from build123d import *

# Parameters (mm, degrees)
EXTRUDE_3_DEPTH     = 18
SKETCH_2_R          = 1.8
CUT_EXTRUDE_1_DEPTH = 17.325
SKETCH_4_R          = 1.75
EXTRUDE_9_DEPTH     = 5
SKETCH_7_W          = 17.320508076
SKETCH_7_H          = 5
EXTRUDE_10_DEPTH    = 25
FILLET_1_R          = 5
FILLET_2_R          = 5
SKETCH_8_R          = 20
EXTRUDE_11_DEPTH    = 3


with BuildPart() as part:
    # 草图1 → 凸台-拉伸3 (new body)
    with BuildSketch(Plane(origin=(0, 0, 0), x_dir=(1, 0, 0), z_dir=(0, 1, 0))):
        Polygon((10, 0), (5, 8.660254038), (-5, 8.660254038), (-10, 0), (-5, -8.660254038), (5, -8.660254038), align=None)
        Polygon((6.985938257, 0), (3.492969129, 6.05), (-3.492969129, 6.05), (-6.985938257, 0), (-3.492969129, -6.05), (3.492969129, -6.05), align=None, mode=Mode.SUBTRACT)
    extrude(amount=-EXTRUDE_3_DEPTH)

    # 草图2 → 切除-拉伸1 (cut)
    with BuildSketch(Plane(origin=(7.5, 0, -4.330127019), x_dir=(-0.5000000000000003, 0, -0.8660254037844386), z_dir=(0.8660254037844386, 0, -0.5000000000000003))):
        with Locations((0, -4.5)):
            Circle(SKETCH_2_R)
    extrude(amount=-CUT_EXTRUDE_1_DEPTH, mode=Mode.SUBTRACT)

    # 草图4 → 凸台-拉伸9 (add)
    with BuildSketch(Plane.XZ.offset(18)):
        Polygon((-10, 0), (5, -8.660254038), (10, 0), (5, 8.660254038), (-5, 8.660254038), align=None)
        with Locations(Location((0, 0, 0), (0, 0, 270))):
            Circle(SKETCH_4_R, mode=Mode.SUBTRACT)
    extrude(amount=EXTRUDE_9_DEPTH)

    # 草图7 → 凸台-拉伸10 (add)
    with BuildSketch(Plane(origin=(-2.5, 0, -4.330127019), x_dir=(-0.8660254037844388, 0, 0.49999999999999983), z_dir=(-0.4999999999999998, 0, -0.8660254037844387))):
        with Locations((0, -20.5)):
            Rectangle(SKETCH_7_W, SKETCH_7_H)
    extrude(amount=EXTRUDE_10_DEPTH)

    # 圆角1
    fillet_1_edges = [part.edges().sort_by_distance(p)[0] for p in [
        (-7.5, -20.5, -30.310889132),
    ]]
    fillet(fillet_1_edges, radius=FILLET_1_R)

    # 圆角2
    fillet_2_edges = [part.edges().sort_by_distance(p)[0] for p in [
        (-22.5, -20.5, -21.650635095),
    ]]
    fillet(fillet_2_edges, radius=FILLET_2_R)

    # 草图8 → 凸台-拉伸11 (add)
    with BuildSketch(Plane.XZ.offset(23)):
        with Locations(Location((-12.169872981, -21.078838325, 0), (0, 0, 85.658906273))):
            Circle(SKETCH_8_R)
    extrude(amount=EXTRUDE_11_DEPTH)


solid = part.part
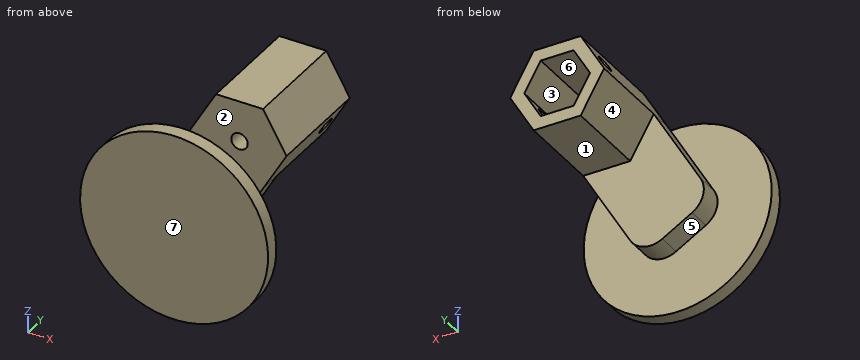
Input: part model. Units: mm. Frame: model coordinates. Face numbers are marked on the shaded views. A direction names the side the tool comes from. Give positions to 0.01 mm unless a question says otherwise; leave off trailing zeros. Write each loop counter-clockwise with the first axis right and the second up, starting at its lowest first coordinate (ties: lowest second). Pieces come first, ordered by that corner, then holes. Notation, with made-up numbers: M 13,35.25 L 64,35.25 A14 cw 64,48.25 Z; hole C 5,-37.5 d4. An arc over 180 degrees is marked long. Write item = value, one per line. Start each with the question number.
1) Draft query along X for the marked faces 5, 6 and 7. Return one class per face: +X half, -X half, draft (parallel to the pull), parting line (faces both ways), or undercut.
2) Reachability of the marked faces 1, 2, 3 and 4 from +Z, -Z, +X, -X, +Y, -Y: full face, straight path, thin tool, end or side. Return the list, or none.
3) First-contact query: pin 1 Ø5 at (x, z) = (-10.5, -22.5) entering from +Y; pin 2 Ø5.5 at (x, y) = (0, -13) entering from -Z; pin 3 Ø1.5 at (y, z) = (-20, -16.5) entering from +X. Flat tips, straight axial feed; report the tip coordinate or a pass-through.
4) Cut plane D-D on x = -26. Return the cut outline in (y, z), then the cut area to 3 significant figures.
5) Cut plane C-C on z = -14. Return the cut outline in (x, y), then the cut area to 3 significant figures.
6) Cut plane A-A on y = -11.5. Return the cut outline in (x, z).
7) Material intervals for line 1 along X through (y, z) = (-19.7, 0); line 2 along Z through (x, y) = (-3, -3.75); line 3 along Y through (x, z) = (-19, -10), sorted ascending. Write a range as [from, to].
8) Cut plane B-B on x = 0. Return the cut outline in (y, z), then the cut area to 3 significant figures.
Solved:
q1.face_5 = -X half
q1.face_6 = undercut
q1.face_7 = draft
q2.face_1 = -Z, +X, -X, +Y
q2.face_2 = +Z, +X, -Y
q2.face_3 = +Y
q2.face_4 = -Z, -X, +Y
q3.pin_1 = -18
q3.pin_2 = -8.66
q3.pin_3 = 0.91
q4.outline = M -26,-35.53 L -23,-35.53 L -23,-6.63 L -26,-6.63 Z
q4.area = 86.7 mm2
q5.outline = M -30.88,-26 L 6.54,-26 L 6.54,-23 L 1.92,-23 L 1.92,-18 L -18.08,-18 L -18.08,-23 L -30.88,-23 Z
q5.area = 212 mm2
q6.outline = M -10,0 L -5,-8.66 L 5,-8.66 L 10,0 L 5,8.66 L -5,8.66 Z; hole M -6.99,0 L -3.49,-6.05 L 3.49,-6.05 L 6.99,0 L 3.49,6.05 L -3.49,6.05 Z
q7.line_1 = [-10, -1.75], [1.75, 10]
q7.line_2 = [-8.66, -6.05], [6.05, 8.66]
q7.line_3 = [-26, -23]
q8.outline = M -26,-36.95 L -23,-36.95 L -23,-17.32 L -18,-17.32 L -18,-8.66 L 0,-8.66 L 0,-6.05 L -18,-6.05 L -18,-1.75 L -23,-1.75 L -23,-5.21 L -26,-5.21 Z; M -23,1.75 L -18,1.75 L -18,6.05 L 0,6.05 L 0,8.66 L -23,8.66 Z
q8.area = 302 mm2
